Here's how the part is built. I have some questions about the finished solid (model axes, mm). Coordinates: 2 decimals unless noted, no trailing zeros. Write each loop counter-clockwise with the first axis right and the second up, starting at its lowest first coordinate (ties: lowest second). Pieces come first, ordered by that corner, then holes.
from build123d import *

# Parameters (mm, degrees)
SKETCH_1_W               = 196
SKETCH_1_H               = 80
EXTRUDE_1_DEPTH          = 5
CUT_EXTRUDE_1_REACH      = 107.967
SKETCH_2_W               = 20
SKETCH_2_H               = 5
PATTERN_LINEAR_1_COUNT   = 3
PATTERN_LINEAR_1_PITCH   = 40
PATTERN_LINEAR_2_COUNT   = 3
PATTERN_LINEAR_2_PITCH   = 40
CUT_EXTRUDE_2_REACH      = 107.967
SKETCH_3_W               = 5
SKETCH_3_H               = 20
MIRROR_2_COPY_1_REACH    = 107.967
MIRROR_2_COPY_1_SKETCH_W = 20
MIRROR_2_COPY_1_SKETCH_H = 5
MIRROR_2_COPY_2_REACH    = 107.967
MIRROR_2_COPY_2_SKETCH_W = 20
MIRROR_2_COPY_2_SKETCH_H = 5
MIRROR_2_COPY_3_REACH    = 107.967
MIRROR_2_COPY_3_SKETCH_W = 20
MIRROR_2_COPY_3_SKETCH_H = 5
MIRROR_2_COPY_4_REACH    = 107.967
MIRROR_2_COPY_4_SKETCH_W = 20
MIRROR_2_COPY_4_SKETCH_H = 5


with BuildPart() as part:
    # 스케치1 → 보스-돌출1 (new body)
    with BuildSketch(Plane(origin=(0, 0, 0), x_dir=(1, 0, 0), z_dir=(0, 1, 0))):
        Rectangle(SKETCH_1_W, SKETCH_1_H)
    extrude(amount=EXTRUDE_1_DEPTH)

    # 스케치2 → 컷-돌출1 (cut, up to next)
    with BuildSketch(Plane(origin=(0, 5, 0), x_dir=(1, 0, 0), z_dir=(0, 1, 0)), mode=Mode.PRIVATE) as cut_extrude_1_sk1:
        with Locations((0, -37.5)):
            Rectangle(SKETCH_2_W, SKETCH_2_H)
    cut_extrude_1_tool1 = extrude(cut_extrude_1_sk1.sketch, amount=-CUT_EXTRUDE_1_REACH, mode=Mode.PRIVATE) & part.part
    cut_extrude_1 = cut_extrude_1_tool1.solids().sort_by_distance((0, 5, 37.5))[0]
    add(cut_extrude_1, mode=Mode.SUBTRACT)

    # 선형 패턴1: 컷-돌출1 ×3
    with Locations(*[(i * PATTERN_LINEAR_1_PITCH, 0, 0) for i in range(1, PATTERN_LINEAR_1_COUNT)]):
        add(cut_extrude_1, mode=Mode.SUBTRACT)

    # 선형 패턴2: 컷-돌출1 ×3
    with Locations(*[(-i * PATTERN_LINEAR_2_PITCH, 0, 0) for i in range(1, PATTERN_LINEAR_2_COUNT)]):
        add(cut_extrude_1, mode=Mode.SUBTRACT)

    # 스케치3 → 컷-돌출2 (cut, up to next)
    with BuildSketch(Plane(origin=(0, 5, 0), x_dir=(1, 0, 0), z_dir=(0, 1, 0)), mode=Mode.PRIVATE) as cut_extrude_2_sk1:
        with Locations((95.5, 0)):
            Rectangle(SKETCH_3_W, SKETCH_3_H)
    cut_extrude_2_tool1 = extrude(cut_extrude_2_sk1.sketch, amount=-CUT_EXTRUDE_2_REACH, mode=Mode.PRIVATE) & part.part
    cut_extrude_2 = cut_extrude_2_tool1.solids().sort_by_distance((95.5, 5, 0))[0]
    add(cut_extrude_2, mode=Mode.SUBTRACT)

    # 대칭 복사2: 컷-돌출1 across plane
    add(cut_extrude_1.mirror(Plane.XY), mode=Mode.SUBTRACT)

    # 대칭 복사2 copy 1 sketch → 대칭 복사2 copy 1 (cut, up to next)
    with BuildSketch(Plane(origin=(40, 5, 0), x_dir=(1, 0, 0), z_dir=(0, 1, 0)), mode=Mode.PRIVATE) as mirror_2_copy_1_sk1:
        with Locations((0, 37.5)):
            Rectangle(MIRROR_2_COPY_1_SKETCH_W, MIRROR_2_COPY_1_SKETCH_H)
    mirror_2_copy_1_tool1 = extrude(mirror_2_copy_1_sk1.sketch, amount=-MIRROR_2_COPY_1_REACH, mode=Mode.PRIVATE) & part.part
    add(mirror_2_copy_1_tool1.solids().sort_by_distance((40, 5, -37.5))[0], mode=Mode.SUBTRACT)

    # 대칭 복사2 copy 2 sketch → 대칭 복사2 copy 2 (cut, up to next)
    with BuildSketch(Plane(origin=(80, 5, 0), x_dir=(1, 0, 0), z_dir=(0, 1, 0)), mode=Mode.PRIVATE) as mirror_2_copy_2_sk1:
        with Locations((0, 37.5)):
            Rectangle(MIRROR_2_COPY_2_SKETCH_W, MIRROR_2_COPY_2_SKETCH_H)
    mirror_2_copy_2_tool1 = extrude(mirror_2_copy_2_sk1.sketch, amount=-MIRROR_2_COPY_2_REACH, mode=Mode.PRIVATE) & part.part
    add(mirror_2_copy_2_tool1.solids().sort_by_distance((80, 5, -37.5))[0], mode=Mode.SUBTRACT)

    # 대칭 복사2 copy 3 sketch → 대칭 복사2 copy 3 (cut, up to next)
    with BuildSketch(Plane(origin=(-40, 5, 0), x_dir=(1, 0, 0), z_dir=(0, 1, 0)), mode=Mode.PRIVATE) as mirror_2_copy_3_sk1:
        with Locations((0, 37.5)):
            Rectangle(MIRROR_2_COPY_3_SKETCH_W, MIRROR_2_COPY_3_SKETCH_H)
    mirror_2_copy_3_tool1 = extrude(mirror_2_copy_3_sk1.sketch, amount=-MIRROR_2_COPY_3_REACH, mode=Mode.PRIVATE) & part.part
    add(mirror_2_copy_3_tool1.solids().sort_by_distance((-40, 5, -37.5))[0], mode=Mode.SUBTRACT)

    # 대칭 복사2 copy 4 sketch → 대칭 복사2 copy 4 (cut, up to next)
    with BuildSketch(Plane(origin=(-80, 5, 0), x_dir=(1, 0, 0), z_dir=(0, 1, 0)), mode=Mode.PRIVATE) as mirror_2_copy_4_sk1:
        with Locations((0, 37.5)):
            Rectangle(MIRROR_2_COPY_4_SKETCH_W, MIRROR_2_COPY_4_SKETCH_H)
    mirror_2_copy_4_tool1 = extrude(mirror_2_copy_4_sk1.sketch, amount=-MIRROR_2_COPY_4_REACH, mode=Mode.PRIVATE) & part.part
    add(mirror_2_copy_4_tool1.solids().sort_by_distance((-80, 5, -37.5))[0], mode=Mode.SUBTRACT)

    # 대칭 복사3: 컷-돌출2 across plane
    add(cut_extrude_2.mirror(Plane(origin=(0, 0, 0), x_dir=(0, 0, 1), z_dir=(1, 0, 0))), mode=Mode.SUBTRACT)


solid = part.part
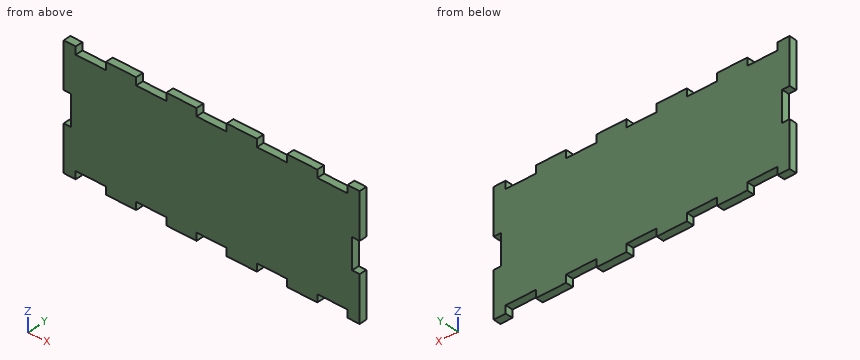
1. I want a section at B-B (x = 47). List the corners of the cut face in (y, z) for me.
2. I want a section at A-A (z = 7). List the corners of the cut face in (x, y) for me.
3. For pin 1 Ø4 at (x, z) = (-7.5, -24) entering from -Y; pin 2 Ø1.5 at (x, y) = (-40, 3.5) entering from -Z; pin 3 Ø2.5 at (x, y) = (4, 1.5) entering from +Z, each with a flat end and sliding along its axis, tell me the tip position at first contact or that it passes through.
4. If I drill on line 1 (Z direction, x = 41, y = 4.6); line 2 (X direction, y = 3.5, z = -3), over which ranges is the centre line in solid material (lowest first)?
Response values:
1. outline: (0, -35) - (5, -35) - (5, 35) - (0, 35) - close
2. outline: (-93, 0) - (93, 0) - (93, 5) - (-93, 5) - close
3. pin 1: stops at y = 0
3. pin 2: stops at z = -35
3. pin 3: stops at z = 35
4. line 1: z = -35 to 35
4. line 2: x = -93 to 93
